Read the model definition and answer for the solid it produces. Units are mm, in the model's axes. Round coordinates to 2 decimals unless told otherwise and drop trailing zeros. Order: outer loops, then holes, each group sorted by start corner. A loop starts at its lowest first (then second) coordinate and runs counter-clockwise, first axis right, second up. Notation, with made-up numbers: M -21.75,0.25 L 23.25,0.25 A11 cw 23.25,8.25 Z; hole C 52.5,50 d8. An arc over 180 degrees is marked long. Answer as CSV lines item,"result".
```python
from build123d import *

# Parameters (mm, degrees)
ESQUISSE1_W        = 5
ESQUISSE1_H        = 5
BOSS_EXTRU_1_DEPTH = 300


with BuildPart() as part:
    # Esquisse1 → Boss.-Extru.1 (new body)
    with BuildSketch(Plane.XY):
        Polygon((0, 9), (7.585786438, 9), (10, 11.414213562), (10, 16), (5.1, 16), (5.1, 20), (20, 20), (20, 5.1), (16, 5.1), (16, 10), (11.414213562, 10), (9, 7.585786438), (9, 0), (9, -7.585786438), (11.414213562, -10), (16, -10), (16, -5.1), (20, -5.1), (20, -20), (5.1, -20), (5.1, -16), (10, -16), (10, -11.414213562), (7.585786438, -9), (0, -9), (-7.585786438, -9), (-10, -11.414213562), (-10, -16), (-5.1, -16), (-5.1, -20), (-20, -20), (-20, -5.1), (-16, -5.1), (-16, -10), (-11.414213562, -10), (-9, -7.585786438), (-9, 0), (-9, 7.585786438), (-11.414213562, 10), (-16, 10), (-16, 5.1), (-20, 5.1), (-20, 20), (-5.1, 20), (-5.1, 16), (-10, 16), (-10, 11.414213562), (-7.585786438, 9), align=None)
        with Locations((15, 15)):
            Rectangle(ESQUISSE1_W, ESQUISSE1_H, mode=Mode.SUBTRACT)
        Polygon((0, 6), (6, 6), (6, 0), (6, -6), (0, -6), (-6, -6), (-6, 0), (-6, 6), align=None, mode=Mode.SUBTRACT)
        with Locations((15, -15)):
            Rectangle(ESQUISSE1_W, ESQUISSE1_H, mode=Mode.SUBTRACT)
        with Locations((-15, -15)):
            Rectangle(ESQUISSE1_W, ESQUISSE1_H, mode=Mode.SUBTRACT)
        with Locations((-15, 15)):
            Rectangle(ESQUISSE1_W, ESQUISSE1_H, mode=Mode.SUBTRACT)
    extrude(amount=BOSS_EXTRU_1_DEPTH)


solid = part.part
```
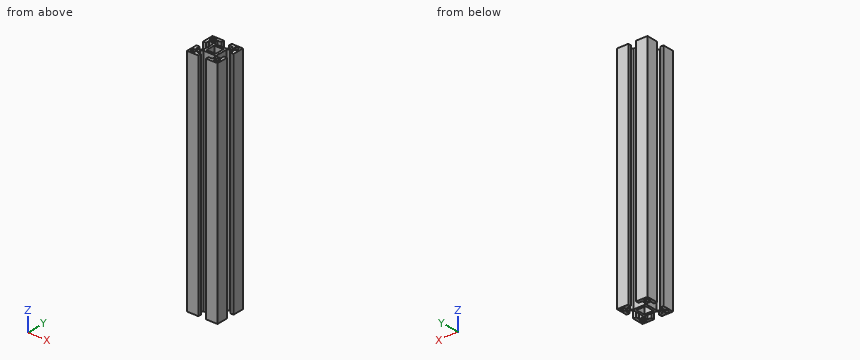
Item 1: Find the intervals of material crossed by probe 1 along Y at (x, z) = (-14, 116); probe 2 along X at (y, z) = (-7, 24); probe 3 along Y at (x, z) = (2, 150), in increasing order. Write a range as [from, to].
Ans:
probe 1,"[-20, -17.5], [-12.5, -10], [10, 12.5], [17.5, 20]"
probe 2,"[-20, -16], [-9, 9], [16, 20]"
probe 3,"[-9, -6], [6, 9]"
Item 2: A flat-ended cylindrical pin translates along its axis: pin 1 (6 mm diameter, centred on x = 0.5, z = 163.5, fed in from -Y). Find the tip coordinate at first contact, or state that the pin passes through.
Ans:
pin 1,"y = -9"
Item 3: A cutting plane is placed at C-C, the plane z = 114.5. Give the number of separate pieces and of enclosed holes in the cut face, and give its area (3 significant figures).
Ans:
separate pieces,"1"
enclosed holes,"5"
area,"656 mm2"
Item 4: A cutting plane is placed at A-A, the plane x = 1. Determine the outline of the cut face in (y, z).
Ans:
outline,"M -9,0 L -6,0 L -6,300 L -9,300 Z; M 6,0 L 9,0 L 9,300 L 6,300 Z"
